Source: CAD feature listing. Evaluate the final solid. Frame: model axes, mm. Face numbers are marked on the shaded views. A direction names the side the tool comes from. Coordinates: 2 decimals unless noted, no trailing zeros. Loops run counter-clockwise (first coordinate to the right, second up) from the corner with the lowest first, then second, coordinate; pieces in that order, holes last. Notation, with made-up numbers: (61.5, -33.5) - (119.5, -33.5) arc R19 cw to (119.5, -14.5) - close; hole circle Ø9 at (51.25, -30.5). An arc over 180 degrees is marked (long way). Use CSV: the item, a comma, the result in double quotes. Start each with the question number.
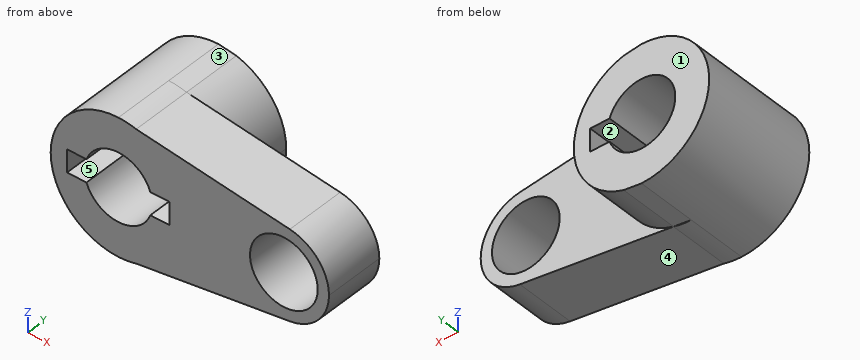
```python
from build123d import *

# Parameters (mm, degrees)
F0_R     = 14.2875
F1_DEPTH = 25.4
F2_DEPTH = 25.146


with BuildPart() as f1:
    # F0 (on Front) → F1 (new body)
    with BuildSketch(Plane.XZ):
        with BuildLine():
            ThreePointArc((7.5208737148, 27.5675004954), (3.7940280931, 28.322005152), (0, 28.575))
            Line((0, 28.575), (7.5208737148, 27.5675004954))
        make_face()
        with BuildLine():
            Line((7.5208737148, -27.5675004954), (0, -28.575))
            ThreePointArc((0, -28.575), (3.7940280931, -28.322005152), (7.5208737148, -27.5675004954))
        make_face()
        with BuildLine():
            Line((72.3621368264, 18.881336768), (7.5208737148, 27.5675004954))
            ThreePointArc((7.5208737148, 27.5675004954), (22.7094648924, 17.3438989071), (28.575, 0))
            ThreePointArc((28.575, 0), (22.7094648924, -17.3438989071), (7.5208737148, -27.5675004954))
            Line((7.5208737148, -27.5675004954), (72.3621368264, -18.881336768))
            ThreePointArc((72.3621368264, -18.881336768), (50.7827847643, 0), (72.3621368264, 18.881336768))
        make_face()
        with BuildLine():
            ThreePointArc((88.8827847643, 0), (84.1695671227, 12.5442884058), (72.3621368264, 18.881336768))
            ThreePointArc((72.3621368264, 18.881336768), (50.7827847643, 0), (72.3621368264, -18.881336768))
            ThreePointArc((72.3621368264, -18.881336768), (84.1695671227, -12.5442884058), (88.8827847643, 0))
        make_face()
        with Locations((69.8327847643, 0)):
            Circle(F0_R, mode=Mode.SUBTRACT)
        with BuildLine():
            Line((7.5208737148, 27.5675004954), (0, 28.575))
            ThreePointArc((0, 28.575), (-28.575, 0), (0, -28.575))
            Line((0, -28.575), (7.5208737148, -27.5675004954))
            ThreePointArc((7.5208737148, -27.5675004954), (22.7094648924, -17.3438989071), (28.575, 0))
            ThreePointArc((28.575, 0), (22.7094648924, 17.3438989071), (7.5208737148, 27.5675004954))
        make_face()
        with BuildLine():
            ThreePointArc((-13.4703841816, 4.7625), (0, 14.2875), (13.4703841816, 4.7625))
            Line((13.4703841816, 4.7625), (21.6587726027, 4.7625))
            Line((21.6587726027, 4.7625), (21.6587726027, -4.7625))
            Line((21.6587726027, -4.7625), (13.4703841816, -4.7625))
            ThreePointArc((13.4703841816, -4.7625), (0, -14.2875), (-13.4703841816, -4.7625))
            Line((-13.4703841816, -4.7625), (-21.6587726027, -4.7625))
            Line((-21.6587726027, -4.7625), (-21.6587726027, 4.7625))
            Line((-21.6587726027, 4.7625), (-13.4703841816, 4.7625))
        make_face(mode=Mode.SUBTRACT)
    extrude(amount=F1_DEPTH)

    # F0 (on Front) → F2 (join)
    with BuildSketch(Plane.XZ):
        with BuildLine():
            Line((7.5208737148, 27.5675004954), (0, 28.575))
            ThreePointArc((0, 28.575), (-28.575, 0), (0, -28.575))
            Line((0, -28.575), (7.5208737148, -27.5675004954))
            ThreePointArc((7.5208737148, -27.5675004954), (22.7094648924, -17.3438989071), (28.575, 0))
            ThreePointArc((28.575, 0), (22.7094648924, 17.3438989071), (7.5208737148, 27.5675004954))
        make_face()
        with BuildLine():
            ThreePointArc((-13.4703841816, 4.7625), (0, 14.2875), (13.4703841816, 4.7625))
            Line((13.4703841816, 4.7625), (21.6587726027, 4.7625))
            Line((21.6587726027, 4.7625), (21.6587726027, -4.7625))
            Line((21.6587726027, -4.7625), (13.4703841816, -4.7625))
            ThreePointArc((13.4703841816, -4.7625), (0, -14.2875), (-13.4703841816, -4.7625))
            Line((-13.4703841816, -4.7625), (-21.6587726027, -4.7625))
            Line((-21.6587726027, -4.7625), (-21.6587726027, 4.7625))
            Line((-21.6587726027, 4.7625), (-13.4703841816, 4.7625))
        make_face(mode=Mode.SUBTRACT)
        with BuildLine():
            ThreePointArc((-13.4703841816, -4.7625), (-14.2875, 0), (-13.4703841816, 4.7625))
            Line((-13.4703841816, 4.7625), (-21.6587726027, 4.7625))
            Line((-21.6587726027, 4.7625), (-21.6587726027, -4.7625))
            Line((-21.6587726027, -4.7625), (-13.4703841816, -4.7625))
        make_face()
    extrude(amount=-F2_DEPTH)


solid = f1.part
```
(1) Section D-D on z = -2.5. Output: boundary loops of the cut face in (x, y).
(2) Ray query, line 1 (X direction, y = -22, z = -8); line 2 (X direction, y = -14.5, z = 4.5); line 3 (Y direction, x = 82.5, z = -9). Return the intervals inside material, ascending. Write a range as [from, to].
(3) Draft query along Z for the marked faces 1, 2 and 3. Return one class per face: released by +Z, released by -Z, zero draft, split by the parting line, or undercut.
(4) Section C-C on x = 62.5. Output: boundary loops of the cut face in (y, z).
(5) Pin query (flat end, axial travel): pin 1 Ø4 at (x, y) = (-18.5, -14.5) entering from -Z; pin 2 Ø7.5 at (y, z) = (2.5, 2) entering from -X (3 decimals); pin 3 Ø9 at (x, z) = (-18.5, 1) entering from -Y; pin 4 Ø4 at (x, y) = (19, 2.5) entering from -Z. Return the tip coordinate at first contact, or that it passes through.
(6) Reachability of the marked faces 4 and 5 from +Z, -Z, +X, -X, +Y, -Y: full face, straight path, thin tool, end or side. Return the list, or none.
(7) Section A-A on y = -7.5. State how many separate pieces and enclosed holes the cut face has, plus the area to 3 significant figures.
Solution:
1,outline,"(-28.47, -25.4) - (-21.66, -25.4) - (-21.66, 0) - (-14.07, 0) - (-14.07, 25.15) - (-28.47, 25.15) - close; (21.66, -25.4) - (55.77, -25.4) - (55.77, 0) - (28.47, 0) - (28.47, 25.15) - (21.66, 25.15) - close; (83.9, -25.4) - (88.72, -25.4) - (88.72, 0) - (83.9, 0) - close"
2,line 1,"x = [-27.43, -11.84], [11.84, 58], [81.67, 87.12]"
2,line 2,"x = [-28.22, -21.66], [21.66, 56.27], [83.39, 88.34]"
2,line 3,"y = [-25.4, 0]"
3,face 1,"zero draft"
3,face 2,"undercut"
3,face 3,"released by +Z"
4,outline,"(-25.4, -20.2) - (0, -20.2) - (0, -12.26) - (-25.4, -12.26) - close; (-25.4, 12.26) - (0, 12.26) - (0, 20.2) - (-25.4, 20.2) - close"
5,pin 1,"stops at z = -23.33"
5,pin 2,"stops at x = -28.575"
5,pin 3,"stops at y = -25.4"
5,pin 4,"stops at z = -22.97"
6,face 4,"-Z, +X, +Y, -Y"
6,face 5,"-Y"
7,separate pieces,"1"
7,enclosed holes,"2"
7,area,"3,770 mm²"
